Here's how the part is built. I have some questions about the finished solid (model axes, mm). Face numbers are marked on the shaded views. A direction names the side the tool comes from. Round coordinates to 2 decimals unless told otherwise and drop trailing zeros. Order: outer loops, then holes, each group sorted by start corner. A loop starts at its lowest first (then second) coordinate and runs counter-clockwise, first axis right, second up.
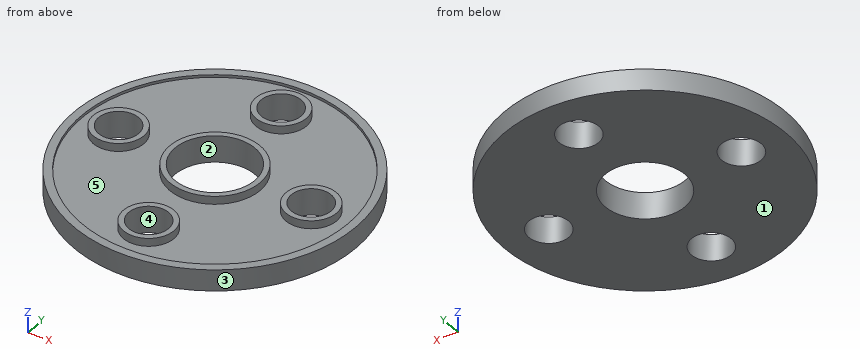
```python
from build123d import *

# Parameters (mm, degrees)
F0_R     = 50
F0_R_2   = 9.5
F0_R_3   = 17
F1_DEPTH = 7
F0_R_4   = 53
F2_DEPTH = 8
F0_R_5   = 7.5
F0_R_6   = 15
F3_DEPTH = 10


with BuildPart() as f1:
    # F0 (on Top) → F1 (new body)
    with BuildSketch(Plane.XY):
        Circle(F0_R)
        with Locations((0, -36)):
            Circle(F0_R_2, mode=Mode.SUBTRACT)
        with Locations((-36, 0)):
            Circle(F0_R_2, mode=Mode.SUBTRACT)
        Circle(F0_R_3, mode=Mode.SUBTRACT)
        with Locations((36, 0)):
            Circle(F0_R_2, mode=Mode.SUBTRACT)
        with Locations((0, 36)):
            Circle(F0_R_2, mode=Mode.SUBTRACT)
    extrude(amount=F1_DEPTH)

    # F0 (on Top) → F2 (join)
    with BuildSketch(Plane.XY):
        Circle(F0_R_4)
        Circle(F0_R, mode=Mode.SUBTRACT)
    extrude(amount=F2_DEPTH)

    # F0 (on Top) → F3 (join)
    with BuildSketch(Plane.XY):
        with Locations((0, 36)):
            Circle(F0_R_2)
        with Locations((0, 36)):
            Circle(F0_R_5, mode=Mode.SUBTRACT)
        with Locations((-36, 0)):
            Circle(F0_R_2)
        with Locations((-36, 0)):
            Circle(F0_R_5, mode=Mode.SUBTRACT)
        with Locations((36, 0)):
            Circle(F0_R_2)
        with Locations((36, 0)):
            Circle(F0_R_5, mode=Mode.SUBTRACT)
        with Locations((0, -36)):
            Circle(F0_R_2)
        with Locations((0, -36)):
            Circle(F0_R_5, mode=Mode.SUBTRACT)
        Circle(F0_R_3)
        Circle(F0_R_6, mode=Mode.SUBTRACT)
    extrude(amount=F3_DEPTH)


solid = f1.part
```
1) If we section it at D-D (y = -40): Write out the boundary of the cut face in (x, z).
2) If we section it at C-C (x = 36): Write out the boundary of the cut face in (y, z), plus the area to 3 significant figures.
3) We'd pull the mould along Y, two halves only. Please class the marked faces 1, 2 and 3: +Y half, -Y half, draft (parallel to the pull), parting line (faces both ways), or undercut.
4) For the marked faces 4 and 5, which set-ups out of +Z, -Z, +X, -X, +Y, -Y let a thin tool reach every point of the face, with its end or its side?
5) If we section it at A-A (x = 0): Give the number of separate pieces and of enclosed holes in the cut face, plus the area to 3 significant figures.
6) I need wall thicknesses on line 1 (Y direction, x = 0, z = 6); line 2 (X direction, y = 1, z = 9.5); line 3 (Y direction, x = -5, z = 4.25). Which ranges of each line are inside material? Lowest first, please.
7) I'm going to push flat-ended pins straight in: pin 1 (19.5 mm diameter, centred on x = -36, y = 0, fed in from +Z); pin 2 (1.5 mm diameter, centred on y = -18.5, z = 5.5, fed in from -X); pin 3 (1 mm diameter, centred on y = -31, z = 9, fed in from +X); pin 4 (9 mm diameter, centred on x = 0, y = 36, fed in from +Z). Where does each tip first touch, or does it pass through?
Solutions:
1. outline: (-34.77, 0) - (-6.34, 0) - (-6.34, 10) - (-8.62, 10) - (-8.62, 7) - (-30, 7) - (-30, 8) - (-34.77, 8) - close; (6.34, 0) - (34.77, 0) - (34.77, 8) - (30, 8) - (30, 7) - (8.62, 7) - (8.62, 10) - (6.34, 10) - close
2. outline: (-38.9, 0) - (-7.5, 0) - (-7.5, 10) - (-9.5, 10) - (-9.5, 7) - (-34.7, 7) - (-34.7, 8) - (-38.9, 8) - close; (7.5, 0) - (38.9, 0) - (38.9, 8) - (34.7, 8) - (34.7, 7) - (9.5, 7) - (9.5, 10) - (7.5, 10) - close
2. area: 460 mm2
3. face 1: draft
3. face 2: undercut
3. face 3: parting line
4. face 4: +Z, -Z
4. face 5: +Z
5. separate pieces: 4
5. enclosed holes: 0
5. area: 364 mm2
6. line 1: y = -53 to -43.5, -28.5 to -15, 15 to 28.5, 43.5 to 53
6. line 2: x = -45.45 to -43.43, -28.57 to -26.55, -16.97 to -14.97, 14.97 to 16.97, 26.55 to 28.57, 43.43 to 45.45
6. line 3: y = -52.76 to -41.59, -30.41 to -14.14, 14.14 to 30.41, 41.59 to 52.76
7. pin 1: stops at z = 10
7. pin 2: stops at x = -49.94
7. pin 3: stops at x = 8.37
7. pin 4: passes through
